Design review of the part built by this model. Coordinates are the model's own, in mm. A direction names the side the tool comes from. Round coordinates to 2 decimals unless told otherwise and drop trailing zeros. Order: outer loops, then holes, each group sorted by start corner. A loop starts at its lowest first (then second) coordinate and runs counter-clockwise, first axis right, second up.
Autodesk Inventor part; units mm, degrees
ref_plane "YZ Plane" through (0, 0, 0) normal (1, 0, 0) x (0, 1, 0)
ref_plane "XZ Plane" through (0, 0, 0) normal (0, 1, 0) x (-1, 0, 0)
ref_plane "XY Plane" through (0, 0, 0) normal (0, 0, 1) x (1, 0, 0)
sketch "Sketch1" plane through (0, 0, 0) normal (0, 0, 1) x (1, 0, 0)
  line L0 (0, 0) -> (110, 0)
  line L1 (110, 0) -> (110, -30)
  line L2 (110, -30) -> (0, -30)
  line L3 (0, -30) -> (0, 0)
  line L4 (10, -30) -> (100, -30)
  line L5 (100, -30) -> (100, -10)
  line L6 (100, -10) -> (10, -10)
  line L7 (10, -10) -> (10, -30)
  point P0 (0, -15)
  point P1 (55, 0)
  dimension "d0" = 110
  dimension "d1" = 30
  dimension "d2" = 10
  dimension "d3" = 10
  dimension "d4" = 10
extrude "Extrusion1" add sketch "Sketch1" along normal blind 10 contours L0 L1 L2 L5 L6 L7 L3
fillet "Fillet1" radius 10 4 edges at (0, 0, 5) (110, 0, 5) (10, -10, 5) (100, -10, 5)
sketch "Sketch2" plane through (0, -30, 0) normal (0, -1, 0) x (1, 0, 0)
  line L0 (0, 0) -> (10, 0)
  line L1 (0, 0) -> (0, 10)
  circle A0 centre (5, 5) radius 2.1
  line L2 (110, 0) -> (110, 10)
  line L3 (100, 0) -> (110, 0)
  circle A1 centre (104.6302, 5) radius 2.1
  point P0 (5, 0)
  point P1 (0, 5)
  point P2 (105, 5)
  point P3 (110, 5)
  dimension "d8" = 5
  dimension "d9" = 5
  dimension "d10" = 4.2
  dimension "d11" = 5
  dimension "d12" = 5
  dimension "d13" = 4.2
extrude "Extrusion2" cut sketch "Sketch2" against normal blind 15
equation "\"d3\" = d2"
equation "\"d5\" = d2"
equation "\"d13\" = d10"
properties part number "side door handle v02"
1) To check wall thickness, follow line 1 along X through (y, z) = (-16.75, 6.25); line 2 along Z through (x, y) = (5, -20); line 3 along Y through (x, z) = (62.5, 4). State the ranges of each line that lie inside material, in increasing order.
Results:
line 1: x = 0 to 3.31, 6.69 to 10.54, 99.46 to 102.94, 106.32 to 110
line 2: z = 0 to 2.9, 7.1 to 10
line 3: y = -10 to 0
2) For faces 1 (the face through (10, -25, 5)), 2 (the face through (5.1, -30, 2.7)), 3 (the face through (5, -15, 5)), list the 3-axis set-ups (+Z, -Z, +X, -X, +Y, -Y) from which the entire face can be reached by the end or side of a thin tool; tool diameter is ignored.
Results:
face 1: +Z, -Z, -Y
face 2: +Z, -Z, +X, -X, -Y
face 3: -Y
3) The part is to be moulded in two halves that separate along Z. For faces 4 (the face through (54, -8, 0)), 5 (the face through (105, -15, 5)), 6 (the face through (110, -20, 5)), 7 (the face through (54, -8, 10)), say which applies: released by +Z, released by -Z, zero draft, split by the parting line, or undercut.
Results:
face 4: released by -Z
face 5: undercut
face 6: zero draft
face 7: released by +Z
4) Take a section at D-D on x = 5. Give the boundary of the cut face in (y, z), plus the area to 3 significant figures.
Results:
outline: (-30, 0) - (-1.34, 0) - (-1.34, 10) - (-30, 10) - (-30, 7.1) - (-15, 7.1) - (-15, 2.9) - (-30, 2.9) - close
area: 224 mm2
5) Take a section at A-A on y = -21.25. Give the boundary of the cut face in (x, z), plus the area to 3 significant figures.
Results:
outline: (0, 0) - (10, 0) - (10, 10) - (0, 10) - close; (100, 0) - (110, 0) - (110, 10) - (100, 10) - close; hole circle Ø4.2 at (5, 5); hole circle Ø4.2 at (104.63, 5)
area: 172 mm2
6) Clearance check with flat-ended pins moving along their axes: P1, Ø1, axis at y = -3.5, z = 6.5, coming from the +X side; P2, Ø5, axis at x = 49, z = 5.5, coming from the -Y side; P3, Ø2, axis at x = 105.5, z = 5, coming from the -Y side. State where each tip first meets the part, or that it passes through.
Results:
P1: stops at x = 108
P2: stops at y = -10
P3: stops at y = -15
7) Take a section at B-B on z = 5. Give the boundary of the cut face in (x, y), plus the area to 3 significant figures.
Results:
outline: (0, -30) - (2.9, -30) - (2.9, -15) - (7.1, -15) - (7.1, -30) - (10, -30) - (10, -20) arc R10 cw to (20, -10) - (90, -10) arc R10 cw to (100, -20) - (100, -30) - (102.53, -30) - (102.53, -15) - (106.73, -15) - (106.73, -30) - (110, -30) - (110, -10) arc R10 ccw to (100, 0) - (10, 0) arc R10 ccw to (0, -10) - close
area: 1,370 mm2
8) Take a section at C-C on y = -13.25. Give the boundary of the cut face in (x, z), plus the area to 3 significant figures.
Results:
outline: (0, 0) - (12.62, 0) - (12.62, 10) - (0, 10) - close; (97.38, 0) - (110, 0) - (110, 10) - (97.38, 10) - close
area: 252 mm2
